from build123d import *

# Parameters (mm, degrees)
BOSS_EXTRUDE1_DEPTH = 0.2
BOSS_EXTRUDE2_DEPTH = 12.58
SKETCH1_8_W         = 162.49
SKETCH1_8_H         = 1
BOSS_EXTRUDE3_DEPTH = 15.58
BOSS_EXTRUDE4_DEPTH = 13.38
BOSS_EXTRUDE5_DEPTH = 2.58
BOSS_EXTRUDE6_DEPTH = 1


with BuildPart() as part:
    # Sketch1 → Boss-Extrude1 (new body)
    with BuildSketch(Plane(origin=(0, 0, 0), x_dir=(1, 0, 0), z_dir=(0, 1, 0))):
        Polygon((-113.845299462, 0), (-110.422649731, -5.92820323), (110.422649731, -5.92820323), (113.845299462, 0), (3.422649731, 191.25763964), (-3.422649731, 191.25763964), align=None)
        Polygon((108.979274058, -3.42820323), (-108.979274058, -3.42820323), (-110.958548116, 0), (-1.979274058, 188.75763964), (1.979274058, 188.75763964), (110.958548116, 0), align=None, mode=Mode.SUBTRACT)
    extrude(amount=BOSS_EXTRUDE1_DEPTH)

    # Sketch1_7 → Boss-Extrude2 (add)
    with BuildSketch(Plane(origin=(0, 0, 0), x_dir=(1, 0, 0), z_dir=(0, 1, 0))):
        Polygon((-95.137949192, 30.402081141), (-96.003974596, 30.902081141), (-113.845299462, 0), (-110.422649731, -5.92820323), (-74.74, -5.92820323), (-74.74, -4.92820323), (-109.845299462, -4.92820323), (-112.690598923, 0), align=None)
        Polygon((-3.422649731, 191.25763964), (-14.758974596, 171.622549002), (-13.892949192, 171.122549002), (-2.845299462, 190.25763964), (2.845299462, 190.25763964), (13.892949192, 171.122549002), (14.758974596, 171.622549002), (3.422649731, 191.25763964), align=None)
        Polygon((109.845299462, -4.92820323), (87.75, -4.92820323), (87.75, -5.92820323), (110.422649731, -5.92820323), (113.845299462, 0), (102.508974596, 19.635090638), (101.642949192, 19.135090638), (112.690598923, 0), align=None)
        Polygon((61.133974596, 91.298692801), (56.133974596, 99.958946839), (55.267949192, 99.458946839), (60.267949192, 90.798692801), align=None)
    extrude(amount=BOSS_EXTRUDE2_DEPTH)

    # Sketch1_8 → Boss-Extrude3 (add)
    with BuildSketch(Plane(origin=(0, 0, 0), x_dir=(1, 0, 0), z_dir=(0, 1, 0))):
        Polygon((-14.758974596, 171.622549002), (-96.003974596, 30.902081141), (-95.137949192, 30.402081141), (-13.892949192, 171.122549002), align=None)
        with Locations((6.505, -5.42820323)):
            Rectangle(SKETCH1_8_W, SKETCH1_8_H)
        Polygon((56.133974596, 99.958946839), (14.758974596, 171.622549002), (13.892949192, 171.122549002), (55.267949192, 99.458946839), align=None)
        Polygon((102.508974596, 19.635090638), (61.133974596, 91.298692801), (60.267949192, 90.798692801), (101.642949192, 19.135090638), align=None)
    extrude(amount=BOSS_EXTRUDE3_DEPTH)

    # Sketch1_9 → Boss-Extrude4 (add)
    with BuildSketch(Plane(origin=(0, 0, 0), x_dir=(1, 0, 0), z_dir=(0, 1, 0))):
        Polygon((-112.113248654, 0), (-110.834936491, -2.214101615), (-109.556624327, -4.42820323), (109.556624327, -4.42820323), (112.113248654, 0), (2.556624327, 189.75763964), (-2.556624327, 189.75763964), align=None)
        Polygon((-110.958548116, 0), (-56.468911087, 94.37881982), (-1.979274058, 188.75763964), (1.979274058, 188.75763964), (110.958548116, 0), (108.979274058, -3.42820323), (-108.979274058, -3.42820323), align=None, mode=Mode.SUBTRACT)
    extrude(amount=-BOSS_EXTRUDE4_DEPTH)

    # Sketch1_10 → Boss-Extrude5 (add)
    with BuildSketch(Plane(origin=(0, 0, 0), x_dir=(1, 0, 0), z_dir=(0, 1, 0))):
        Polygon((-95.137949192, 30.402081141), (-96.003974596, 30.902081141), (-113.845299462, 0), (-110.422649731, -5.92820323), (-74.74, -5.92820323), (-74.74, -4.92820323), (-109.845299462, -4.92820323), (-112.690598923, 0), align=None)
        Polygon((-3.422649731, 191.25763964), (-14.758974596, 171.622549002), (-13.892949192, 171.122549002), (-2.845299462, 190.25763964), (2.845299462, 190.25763964), (13.892949192, 171.122549002), (14.758974596, 171.622549002), (3.422649731, 191.25763964), align=None)
        Polygon((109.845299462, -4.92820323), (87.75, -4.92820323), (87.75, -5.92820323), (110.422649731, -5.92820323), (113.845299462, 0), (102.508974596, 19.635090638), (101.642949192, 19.135090638), (112.690598923, 0), align=None)
        Polygon((61.133974596, 91.298692801), (56.133974596, 99.958946839), (55.267949192, 99.458946839), (60.267949192, 90.798692801), align=None)
    extrude(amount=-BOSS_EXTRUDE5_DEPTH)

    # Sketch1_11 → Boss-Extrude6 (add)
    with BuildSketch(Plane(origin=(0, 0, 0), x_dir=(1, 0, 0), z_dir=(0, 1, 0))):
        Polygon((-109.556624327, -4.42820323), (-110.834936491, -2.214101615), (-112.113248654, 0), (-2.556624327, 189.75763964), (2.556624327, 189.75763964), (112.113248654, 0), (109.556624327, -4.42820323), align=None)
        Polygon((-108.979274058, -3.42820323), (-110.958548116, 0), (-56.468911087, 94.37881982), (-1.979274058, 188.75763964), (1.979274058, 188.75763964), (110.958548116, 0), (108.979274058, -3.42820323), align=None, mode=Mode.SUBTRACT)
    extrude(amount=BOSS_EXTRUDE6_DEPTH)


solid = part.part
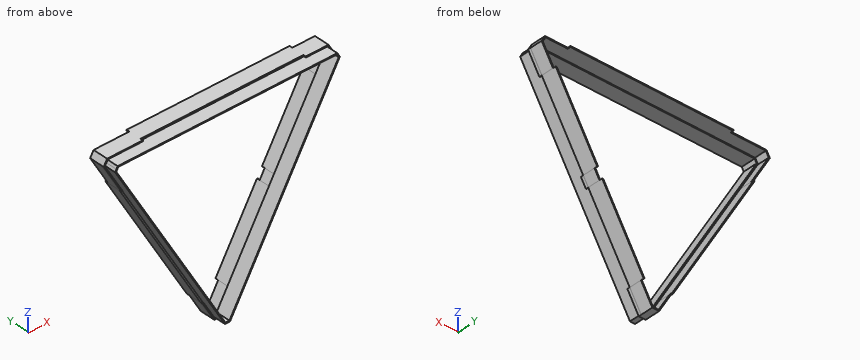
Check sheet for the modelled part. Datum: model origin and axes. Units: mm. Coordinates: 2 decimals unless noted, no trailing zeros. Loops run counter-clockwise (first coordinate to the right, second up) from the corner with the lowest first, then second, coordinate; pieces in that order, holes last. Notation, with made-up numbers: (-25.5, 28) -> (17.5, 28) arc R27 cw to (17.5, 44) -> close; hole circle Ø10 at (51.25, -25.75). An arc over 180 degrees is marked (long way). Answer in a Markdown table with one row per item.
1. Sectioned sample at C-C, the plane x = -88.5. Record the boundary of the cut face in (y, z).
Check values:
| item | result |
|---|---|
| outline | (-13.38, -40.9) -> (0, -40.9) -> (0, -43.9) -> (15.58, -43.9) -> (15.58, -41.9) -> (0.2, -41.9) -> (0.2, -40.9) -> (1, -40.9) -> (1, -38.9) -> (-13.38, -38.9) -> close; (-13.38, 3.43) -> (1, 3.43) -> (1, 4.43) -> (0.2, 4.43) -> (0.2, 4.93) -> (12.58, 4.93) -> (12.58, 5.93) -> (-2.58, 5.93) -> (-2.58, 4.93) -> (0, 4.93) -> (0, 4.43) -> (-13.38, 4.43) -> close |
2. Sectioned sample at D-D, the plane y = -6. Record the boundary of the cut face in (x, z).
Check values:
| item | result |
|---|---|
| outline | (-112.11, 0) -> (-2.56, -189.76) -> (2.56, -189.76) -> (112.11, 0) -> (109.56, 4.43) -> (-109.56, 4.43) -> close; hole (-110.96, 0) -> (-1.98, -188.76) -> (1.98, -188.76) -> (110.96, 0) -> (108.98, 3.43) -> (-108.98, 3.43) -> close |
3. Material ranges on line 1 along Z through (x, y) = (95.5, -2.25) (3 decimals); line 2 along Z through (x, y) = (-15, 0.5); line 3 along X through (y, z) = (0.25, -74.5), recorded low to high. Write a range as [from, to].
Check values:
| item | result |
|---|---|
| line 1 | z = [-28.775, -26.775], [3.428, 4.428], [4.928, 5.928] |
| line 2 | z = [-171.21, -169.21], [-168.21, -166.21], [3.43, 4.43], [4.93, 5.93] |
| line 3 | x = [-70.83, -69.68], [-69.1, -67.95], [67.95, 69.1], [69.68, 70.83] |
4. Go/stop test with flat-tipped pins: pin 1 (0.8 mm diameter, centred on y = -1.5, z = 5.5, fed in from -X); pin 2 (5.5 mm diameter, centred on x = 0.5, y = -3.5, fed in from -Z); pin 3 (2 mm diameter, centred on y = -8.5, z = -103.5, fed in from +X); pin 4 (2 mm diameter, centred on x = -99, y = -1.5, fed in from -Z). Record where each tip stops, or that it passes through.
Check values:
| item | result |
|---|---|
| pin 1 | stops at x = -110.9 |
| pin 2 | stops at z = -191.26 |
| pin 3 | stops at x = 52.93 |
| pin 4 | stops at z = -27.44 |
5. Sectioned sample at A-A, the plane y = 9.75. Record the boundary of the cut face in (x, z), then the cut area to 3 significant figures.
Check values:
| item | result |
|---|---|
| outline | (-113.85, 0) -> (-3.42, -191.26) -> (3.42, -191.26) -> (113.85, 0) -> (110.42, 5.93) -> (-110.42, 5.93) -> close; hole (-112.69, 0) -> (-2.85, -190.26) -> (2.85, -190.26) -> (112.69, 0) -> (109.85, 4.93) -> (-109.85, 4.93) -> close |
| area | 680 mm2 |
6. Sectioned sample at B-B, the plane z = -121. Record the boundary of the cut face in (x, y), then the cut area to 3 significant figures.
Check values:
| item | result |
|---|---|
| outline | (-43.99, 0) -> (-42.25, 0) -> (-42.25, -13.38) -> (-41.1, -13.38) -> (-41.1, 1) -> (-42.25, 1) -> (-42.25, 0.2) -> (-42.83, 0.2) -> (-42.83, 15.58) -> (-43.99, 15.58) -> close; (41.1, -13.38) -> (42.25, -13.38) -> (42.25, 0) -> (43.99, 0) -> (43.99, 15.58) -> (42.83, 15.58) -> (42.83, 0.2) -> (42.25, 0.2) -> (42.25, 1) -> (41.1, 1) -> close |
| area | 69.4 mm2 |
